Part model, mm, in its own coordinate system. A direction names the side the tool comes from. Round coordinates to 2 decimals unless told otherwise and drop trailing zeros. Loops run counter-clockwise (first coordinate to the right, second up) from the corner with the lowest first, then second, coordinate; pieces in that order, holes last. Notation, with made-up numbers: (80, 37) -> (117, 37) arc R15 cw to (117, 46) -> close; hole circle Ø6 at (69, 77.25). An arc over 180 degrees is marked (long way). Answer as a JSON object with one key per item and string values. Group by question number.
from build123d import *

# Parameters (mm, degrees)
F0_W     = 21
F0_H     = 21
F0_W_2   = 15.5
F0_H_2   = 15.5
F0_W_3   = 12.5
F0_H_3   = 12.5
F1_DEPTH = 2
F2_DEPTH = 7


with BuildPart() as f1:
    # F0 (on Top) → F1 (new body)
    with BuildSketch(Plane.XY):
        Rectangle(F0_W, F0_H)
        Rectangle(F0_W_2, F0_H_2, mode=Mode.SUBTRACT)
        Rectangle(F0_W_2, F0_H_2)
        Rectangle(F0_W_3, F0_H_3, mode=Mode.SUBTRACT)
        Rectangle(F0_W_3, F0_H_3)
    extrude(amount=-F1_DEPTH)

    # F0 (on Top) → F2 (join)
    with BuildSketch(Plane.XY):
        Rectangle(F0_W, F0_H)
        Rectangle(F0_W_2, F0_H_2, mode=Mode.SUBTRACT)
        Rectangle(F0_W_3, F0_H_3)
    extrude(amount=F2_DEPTH)


solid = f1.part
Item 1: Band-saw the part on A-A, the plane z = 3. List the corners of the cut face in (x, y).
Item 2: Band-saw the part on B-B, the plane y = 3.25. List the corners of the cut face in (x, z), plus the area to 3 significant figures.
Item 3: Which spindle directions (+Z, -Z, +X, -X, +Y, -Y) get a long thin tool onto all of the face, cutting with end or side? Do faces 1 (the face through (0, 0, 7)), 2 (the face through (0, 6.25, 3)). Say none if no direction does.
Item 4: Band-saw the part on C-C, the plane x = -7.25. List the corners of the cut face in (y, z).
Item 5: Two-plate mould, pull along X, no slides. Class faces 3 (the face through (0, 0, -2)), 4 (the face through (-7, 0, 0)), 5 (the face through (10.5, 0, 2)): pulls with the +X half, pulls with the -X half, needs draft (parallel to the pull), parting line crosses it, or undercut.
Item 6: Drill centre lines: line 1 (Y direction, x = 4.5, z = 0.25); line 2 (Z direction, x = -6.75, y = 3.5). Where is each one in solid material? Low to high.
Entries:
{
 "1": {"outline": "(-10.5, -10.5) -> (10.5, -10.5) -> (10.5, 10.5) -> (-10.5, 10.5) -> close; (-6.25, -6.25) -> (6.25, -6.25) -> (6.25, 6.25) -> (-6.25, 6.25) -> close; hole (-7.75, -7.75) -> (7.75, -7.75) -> (7.75, 7.75) -> (-7.75, 7.75) -> close"},
 "2": {"outline": "(-10.5, -2) -> (10.5, -2) -> (10.5, 7) -> (7.75, 7) -> (7.75, 0) -> (6.25, 0) -> (6.25, 7) -> (-6.25, 7) -> (-6.25, 0) -> (-7.75, 0) -> (-7.75, 7) -> (-10.5, 7) -> close", "area": "168 mm²"},
 "3": {"face 1": "+Z, +X, -X, +Y, -Y", "face 2": "+Z"},
 "4": {"outline": "(-10.5, -2) -> (10.5, -2) -> (10.5, 7) -> (7.75, 7) -> (7.75, 0) -> (-7.75, 0) -> (-7.75, 7) -> (-10.5, 7) -> close"},
 "5": {"face 3": "needs draft", "face 4": "undercut", "face 5": "pulls with the +X half"},
 "6": {"line 1": "-10.5 to -7.75, -6.25 to 6.25, 7.75 to 10.5", "line 2": "-2 to 0"}
}
